Part print with two shaded views. Sizes in mm from the minimum x, y, z corner. A direction names the side the tool comes from. Give positions to 0.01 mm unless a question says otherwise; leave off trailing zeros. Order: outer loops, then holes, each group sorted by start corner. A loop starts at its lowest first (then second) coordinate and runs counter-clockwise, first axis right, second up. Notation, with made-up numbers: (87, 10) -> (94, 10) arc R16 cw to (94, 20) -> close; hole circle Ø8 at (0.25, 74). An arc over 180 degrees is marked (long way). Answer as CSV lines item,"result".
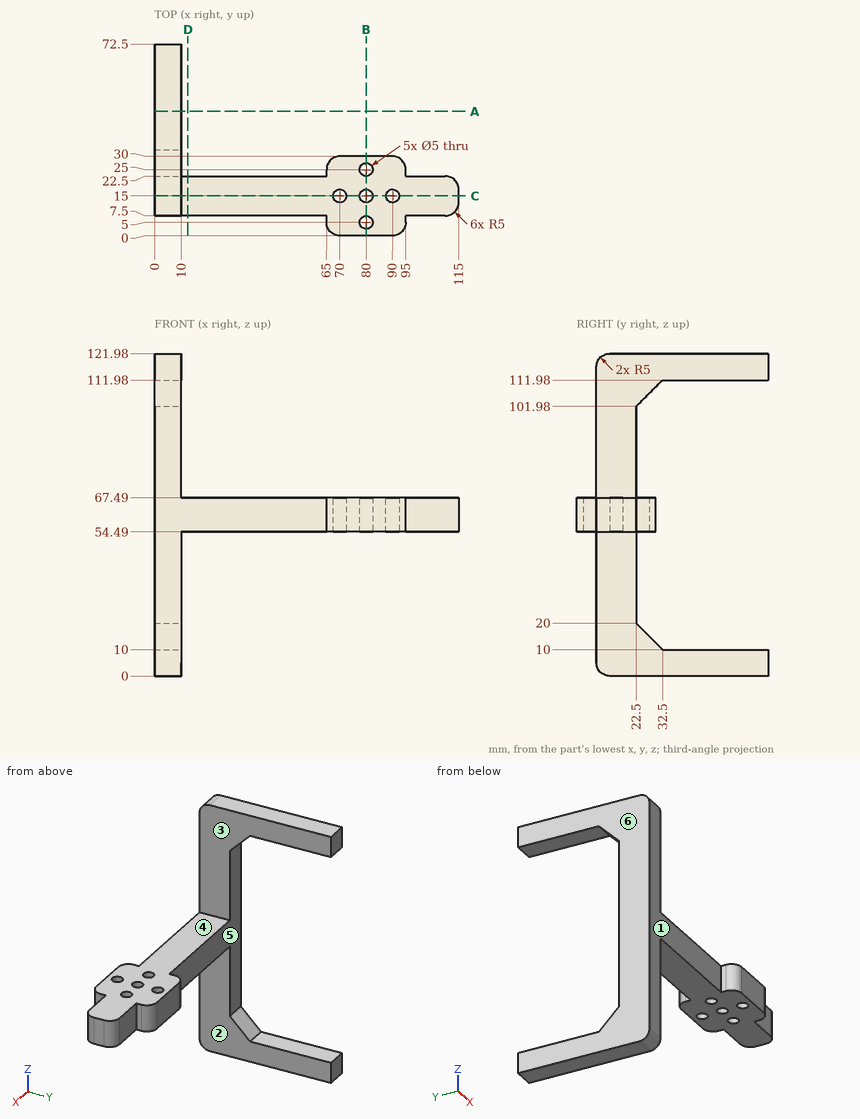
1) Wall check: line 1 along Y through (x, z) = (80, 63.75); line 2 along X through (y, z) = (20, 111); line 3 along X through (y, z) = (12, 65.5). Give the ranges that are in metal, low to high. Write a range as [from, to].
Data:
line 1,"y = [0, 2.5], [7.5, 12.5], [17.5, 22.5], [27.5, 30]"
line 2,"x = [0, 10]"
line 3,"x = [0, 114.97]"
2) Pull direction Z, two halves, no side cores. Call the marked faces 4, 5 and 6: pulls with the +Z half, pulls with the -Z half, needs draft (parallel to the pull), parting line crosses it, or undercut.
Data:
face 4,"pulls with the +Z half"
face 5,"undercut"
face 6,"needs draft"
3) Band-saw the part on A-A, the plane y = 47. Write the cut outline in (x, z).
Data:
outline,"(0, 0) -> (10, 0) -> (10, 10) -> (0, 10) -> close; (0, 111.98) -> (10, 111.98) -> (10, 121.98) -> (0, 121.98) -> close"
4) Pin check, flat tips, straight feed: P1, Ø5, axis at x = 11.5, z = 50, coming from the -Y side; P2, Ø0.8, axis at y = 24, z = 61, coming from the +X side; P3, Ø1.2, axis at y = 6.5, z = 58, coming from the -X side. Stop position of each tip, or through.
Data:
P1,"stops at y = 7.5"
P2,"stops at x = 95"
P3,"stops at x = 65"
5) Band-saw the part on D-D, the plane x = 12.5. Write the cut outline in (y, z), then the cut area to 3 significant figures.
Data:
outline,"(7.5, 54.49) -> (22.5, 54.49) -> (22.5, 67.49) -> (7.5, 67.49) -> close"
area,"195 mm2"
6) Band-saw the part on C-C, the plane y = 15. Write the cut outline in (x, z).
Data:
outline,"(0, 0) -> (10, 0) -> (10, 54.49) -> (67.5, 54.49) -> (67.5, 67.49) -> (10, 67.49) -> (10, 121.98) -> (0, 121.98) -> close; (72.5, 54.49) -> (77.5, 54.49) -> (77.5, 67.49) -> (72.5, 67.49) -> close; (82.5, 54.49) -> (87.5, 54.49) -> (87.5, 67.49) -> (82.5, 67.49) -> close; (92.5, 54.49) -> (115, 54.49) -> (115, 67.49) -> (92.5, 67.49) -> close"
7) Which spindle directions (+Z, -Z, +X, -X, +Y, -Y) get a long thin tool onto all of the face, cutting with end or side? Do the marked faces 1, 2 and 3. Say none if no direction does.
Data:
face 1,"+Z, -Z, -X, -Y"
face 2,"-Z, +X, +Y, -Y"
face 3,"+Z, +X, +Y, -Y"
8) Band-saw the part on B-B, the plane x = 80. Write the cut outline in (y, z), then the cut area to 3 significant figures.
Data:
outline,"(0, 54.49) -> (2.5, 54.49) -> (2.5, 67.49) -> (0, 67.49) -> close; (7.5, 54.49) -> (12.5, 54.49) -> (12.5, 67.49) -> (7.5, 67.49) -> close; (17.5, 54.49) -> (22.5, 54.49) -> (22.5, 67.49) -> (17.5, 67.49) -> close; (27.5, 54.49) -> (30, 54.49) -> (30, 67.49) -> (27.5, 67.49) -> close"
area,"195 mm2"
